Autodesk Inventor part; units mm, degrees
ref_plane "YZ Plane" through (0, 0, 0) normal (1, 0, 0) x (0, 1, 0)
ref_plane "XZ Plane" through (0, 0, 0) normal (0, 1, 0) x (-1, 0, 0)
ref_plane "XY Plane" through (0, 0, 0) normal (0, 0, 1) x (1, 0, 0)
sketch "Sketch1" plane through (0, 0, 0) normal (0, 0, 1) x (1, 0, 0)
  arc A0 (11.9, 11.9) -> (-11.9, 11.9) centre (0, 11.9) ccw
  line L0 (-11.9, 11.9) -> (-11.9, 0)
  line L1 (-11.9, 0) -> (11.9, 0)
  line L2 (11.9, 0) -> (11.9, 11.9)
  circle A1 centre (0, 11.9) radius 4.75
  point P0 (0, 0)
  dimension "d0" = 11.9
  dimension "d1" = 180
  dimension "d2" = 11.9
  dimension "d3" = 9.5
  dimension "d4" = 23.8
  dimension "d5" = 0
extrude "Extrusion1" add sketch "Sketch1" along normal blind 1.75 and the other way blind 9.37
sketch "Sketch2" plane through (-11.9, 0, 1.75) normal (0, -1, 0) x (1, 0, 0)
  circle A0 centre (4.28, -1.75) radius 0.4065
  circle A1 centre (19.52, -1.75) radius 0.4065
  circle A2 centre (11.9, -9.37) radius 0.4065
  point P0 (11.9, -1.75)
  dimension "d10" = 0.813
  dimension "d11" = 0.813
  dimension "d12" = 15.24
  dimension "d13" = 7.62
  dimension "d14" = 0.813
  dimension "d15" = 7.62
extrude "Extrusion2" add sketch "Sketch2" along normal blind 6
equation "\"d11\" = d10"
equation "\"d14\" = d10"
properties part number "AC1015"
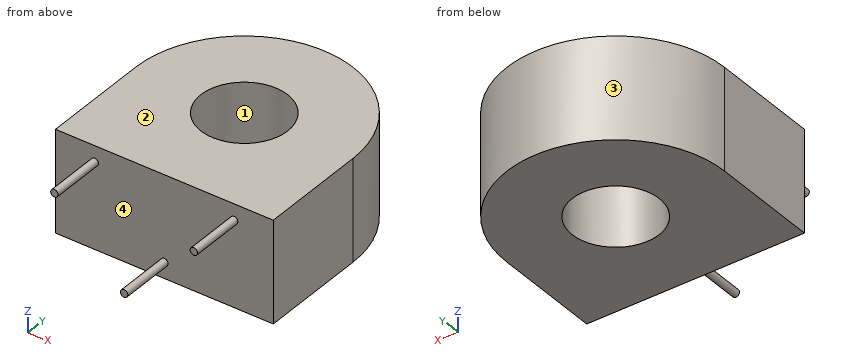
The listing builds one solid part. Answer for the finished solid, in the listing's coordinates (mm). Face numbers are marked on the shaded views. Give positions to 0.01 mm unless a question says otherwise; leave off trailing zeros. Loops run counter-clockwise (first coordinate to the right, second up) from the corner with the lowest first, then second, coordinate; pieces in that order, holes last. Notation, with made-up numbers: M 36,86.5 L 56,86.5 A11 cw 56,97.5 Z; hole C -4,71 d8. An arc over 180 degrees is marked long. One line per item, written item: value.
1. Find the intervals of material crossed by probe 1 along Y at (x, z) = (0, -5.5); probe 2 along Y at (x, z) = (-3.25, -9); probe 3 along X at (y, z) = (11, -0.25), in increasing order.
Found:
probe 1: 0 to 7.15, 16.65 to 23.8
probe 2: 0 to 8.44, 15.36 to 23.35
probe 3: -11.9 to -4.66, 4.66 to 11.9
2. Section C-C on z = -5 is taken. Determine the outline of the cut face in (x, y), plus the area to 3 significant figures.
Found:
outline: M -11.9,0 L 11.9,0 L 11.9,11.9 A11.9 ccw -11.9,11.9 Z; hole C 0,11.9 d9.5
area: 435 mm^2
3. Section A-A on y = 8 is taken. Determine the outline of the cut face in (x, z).
Found:
outline: M -11.9,-9.37 L -2.71,-9.37 L -2.71,1.75 L -11.9,1.75 Z; M 2.71,-9.37 L 11.9,-9.37 L 11.9,1.75 L 2.71,1.75 Z
4. Section B-B on x = 4.25 is taken. Determine the outline of the cut face in (y, z), plus the area to 3 significant figures.
Found:
outline: M 0,-9.37 L 9.78,-9.37 L 9.78,1.75 L 0,1.75 Z; M 14.02,-9.37 L 23.02,-9.37 L 23.02,1.75 L 14.02,1.75 Z
area: 209 mm^2
5. Each of these flat-tipped pins is pushed along its axis until it touches: P1, Ø1.5, axis at x = 3.5, y = -1, coming from the +Z side; P2, Ø1, axis at x = -7, z = -8, coming from the +Y side; P3, Ø5, axis at x = -1.5, z = -4.5, coming from the -Y side; P4, Ø1.5, axis at x = -4, z = 0.5, coming from the +Y side. Where does it stop, or does it pass through?
Found:
P1: through
P2: y = 21.87
P3: y = 0
P4: y = 23.35
6. Section D-D on x = 7.62 is taken. Determine the outline of the cut face in (y, z), plus the area to 3 significant figures.
Found:
outline: M -6,-0.41 L 0,-0.41 L 0,-9.37 L 21.04,-9.37 L 21.04,1.75 L 0,1.75 L 0,0.41 L -6,0.41 Z
area: 239 mm^2
7. For a pull along Y with two mould halves and no side action, classify the marked faces 1, 2, 3 and 4 as pulls with the +Y half, pulls with the -Y half, needs draft (parallel to the pull), parting line crosses it, or undercut.
Found:
face 1: undercut
face 2: needs draft
face 3: pulls with the +Y half
face 4: pulls with the -Y half
